Part model, mm, in its own coordinate system. A direction names the side the tool comes from. Give positions to 0.01 mm unless a question says otherwise; leave off trailing zeros. Order: outer loops, then holes, each group sorted by start corner. A loop starts at its lowest first (then second) coordinate and runs counter-clockwise, first axis right, second up. Notation, with made-up numbers: (40.25, 20) - (84.25, 20) arc R5 ccw to (84.25, 25) - close; hole circle Ø7 at (48.5, 75). An arc over 180 degrees is marked (long way). One line per item, written item: value.
Autodesk Inventor part; units mm, degrees
ref_plane "to_dummy_R_XY" through (0, 0, 0) normal (0, 0, 1) x (1, 0, 0)
ref_plane "to_dummy_R_YZ" through (0, 0, 0) normal (1, 0, 0) x (0, 1, 0)
ref_plane "to_dummy_R_ZX" through (0, 0, 0) normal (0, 1, 0) x (0, 0, 1)
sketch "Sketch_1" plane through (0, 0, 0) normal (1, 0, 0) x (0, 1, 0)
  line L0 (30.226, 0) -> (1.27, 0)
  arc A0 (1.27, 0) -> (0, -1.27) centre (1.27, -1.27) ccw
  line L1 (0, -1.27) -> (0, -20.7518)
  line L2 (0, -20.7518) -> (3.0378, -20.7518)
  line L3 (3.0378, -20.7518) -> (3.0378, -4.3078)
  arc A1 (4.3078, -3.0378) -> (3.0378, -4.3078) centre (4.3078, -4.3078) ccw
  line L4 (4.3078, -3.0378) -> (30.226, -3.0378)
  line L5 (30.226, -3.0378) -> (30.226, 0)
extrude "Extrusion1" add sketch "Sketch_1" along normal blind 28.575
sketch "Sketch_2" plane through (0, 0, 0) normal (0, 0, 1) x (1, 0, 0)
  line L0 (-28.575, -30.226) -> (42.8625, -30.226)
  line L1 (42.8625, -30.226) -> (42.8625, 45.339)
  line L2 (42.8625, 45.339) -> (-28.575, 45.339)
  line L3 (-28.575, 45.339) -> (-28.575, -30.226)
  line L4 (0, 0) -> (28.575, 0)
  line L5 (28.575, 0) -> (28.575, 6.35)
  line L6 (28.575, 6.35) -> (14.4921, 26.7427)
  arc A0 (14.4921, 26.7427) -> (0, 22.225) centre (7.9502, 22.225) ccw
  line L7 (0, 22.225) -> (0, 0)
extrude "Extrusion2" cut sketch "Sketch_2" against normal blind 20.7518
sketch "Sketch3" plane through (0, 1.27, 0) normal (0, 0, 1) x (1, 0, 0)
  point P0 (7.9502, 20.955)
hole "Hole1" at (7.9502, 22.225, 0) direction (0, 0, -1) diameter 6.4198 depth 3.0378
sketch "Sketch4" plane through (0, 0, -20.7518) normal (0, -1, 0) x (1, 0, 0)
  point P0 (4.7625, 9.5631)
hole "Hole2" at (4.7625, 0, -11.1887) direction (0, 1, 0) diameter 6.858 depth 3.0378
sketch "Sketch5" plane through (0, 0, -20.7518) normal (0, -1, 0) x (1, 0, 0)
  point P0 (23.8125, 9.5631)
hole "Hole3" at (23.8125, 0, -11.1887) direction (0, 1, 0) diameter 6.858 depth 3.0378
sketch "Sketch_6" plane through (0, 0, 0) normal (0, 1, 0) x (-1, 0, 0)
  line L0 (0, -14.6177) -> (0, -7.7597)
  line L1 (0, -7.7597) -> (-4.7625, -7.7597)
  line L2 (-4.7625, -7.7597) -> (-4.7625, -14.6177)
  line L3 (-4.7625, -14.6177) -> (0, -14.6177)
sketch "Sketch_7" plane through (0, 0, 0) normal (0, 1, 0) x (-1, 0, 0)
  line L0 (-23.8125, -14.6177) -> (-23.8125, -7.7597)
  line L1 (-23.8125, -7.7597) -> (-28.575, -7.7597)
  line L2 (-28.575, -7.7597) -> (-28.575, -14.6177)
  line L3 (-28.575, -14.6177) -> (-23.8125, -14.6177)
extrude "Extrusion3" cut sketch "Sketch_6" along normal blind 3.0378
extrude "Extrusion4" cut sketch "Sketch_7" along normal blind 3.0378
sketch "Sketch_8" plane through (0, 0, 0) normal (0, 1, 0) x (-1, 0, 0)
  line L0 (0, -31.1277) -> (0, -19.4818)
  arc A0 (-1.27, -20.7518) -> (0, -19.4818) centre (-1.27, -19.4818) ccw
  line L1 (-1.27, -20.7518) -> (-27.305, -20.7518)
  arc A1 (-28.575, -19.4818) -> (-27.305, -20.7518) centre (-27.305, -19.4818) ccw
  line L2 (-28.575, -19.4818) -> (-28.575, -31.1277)
  line L3 (-28.575, -31.1277) -> (0, -31.1277)
extrude "Extrusion5" cut sketch "Sketch_8" along normal blind 3.0378
ref_plane "to_dummy_R_XY" through (0, 0, 0) normal (0, 0, 1) x (1, 0, 0)
ref_plane "to_dummy_R_YZ" through (0, 0, 0) normal (1, 0, 0) x (0, 1, 0)
ref_plane "to_dummy_R_ZX" through (0, 0, 0) normal (0, 1, 0) x (0, 0, 1)
ref_plane "to_pin_R_XY" through (7.9502, 22.225, 0) normal (0, 0, 1) x (1, 0, 0)
ref_plane "to_pin_R_YZ" through (7.9502, 22.225, 0) normal (1, 0, 0) x (0, 1, 0)
ref_plane "to_pin_R_ZX" through (7.9502, 22.225, 0) normal (0, 1, 0) x (0, 0, 1)
properties part number "D-9966"
1) Cut at D-D, the plane y = 7. Give the cut face in (x, z), then the cut area to 3 significant figures.
Outcome:
outline: (0, -3.04) - (28.13, -3.04) - (28.13, 0) - (0, 0) - close
area: 85.4 mm^2
2) Which spindle directions (+Z, -Z, +X, -X, +Y, -Y) get a long thin tool onto all of the face, cutting with end or side? Do faces 5 (the flat face through (11, 14, -3.038)), 6 (the flat face through (0, 1, -17)), 7 (the flat face through (2, 1, -7.76)), 8 (the flat face through (26, 1, -7.76)). Say none if no direction does.
Outcome:
face 5: -Z, +X, -X, +Y
face 6: +Z, -Z, -X, +Y, -Y
face 7: -X, +Y, -Y
face 8: +X, +Y, -Y
3) Drill centre lines: line 1 along Z through (x, y) = (26.75, 3); line 2 along Y through (x, z) = (26.5, -6); line 3 along Z through (x, y) = (25.75, 4.5). Where is each one in solid material? Low to high. Write a range as from..to.
Outcome:
line 1: z = -20.75..-14.62, -7.76..0
line 2: y = 0..3.04
line 3: z = -3.04..0
4) Cut at B-B, the plane x = 5.25. Give the cut face in (y, z), then the cut area to 3 significant figures.
Outcome:
outline: (0, -20.75) - (3.04, -20.75) - (3.04, -14.58) - (0, -14.58) - close; (0, -7.79) - (3.04, -7.79) - (3.04, -4.31) arc R1.27 cw to (4.31, -3.04) - (20.49, -3.04) - (20.49, 0) - (1.27, 0) arc R1.27 ccw to (0, -1.27) - close; (23.96, -3.04) - (29.7, -3.04) - (29.7, 0) - (23.96, 0) - close
area: 113 mm^2
5) Cut at A-A, the plane x = 8.75. Give the cut face in (y, z), then the cut area to 3 significant figures.
Outcome:
outline: (0, -20.75) - (3.04, -20.75) - (3.04, -4.31) arc R1.27 cw to (4.31, -3.04) - (19.12, -3.04) - (19.12, 0) - (1.27, 0) arc R1.27 ccw to (0, -1.27) - close; (25.33, -3.04) - (30.13, -3.04) - (30.13, 0) - (25.33, 0) - close
area: 126 mm^2
6) Mould opens along Z. For faces 1 (the cylindrical face through (20.384, 1.54, -11.264)), 2 (the flat face through (14, 1, -20.752)), 3 (the flat face through (26, 1, -14.618)), 4 (the flat face through (14, 3.038, -13)) say: released by +Z, released by -Z, zero draft, split by the parting line, or undercut.
Outcome:
face 1: undercut
face 2: released by -Z
face 3: undercut
face 4: zero draft
7) Pin check, flat tips, straight feed: pin 1 (10 mm diameter, centred on x = 18, y = 16, fed in from +Z); pin 2 (8 mm diameter, centred on x = 21.5, y = 11.5, fed in from -Z); pin 3 (8 mm diameter, centred on x = 16.5, z = -12, fed in from +Y). Stop position of each tip, or through.
Outcome:
pin 1: stops at z = 0
pin 2: stops at z = -3.04
pin 3: stops at y = 3.04
8) Cut at C-C, the plane z = -17. Give the cut face in (x, y) (3 decimals).
Outcome:
outline: (0, 0) - (28.575, 0) - (28.575, 3.038) - (0, 3.038) - close
